Geometry check sheet. Reference: drawing and pictorial views, mm from the part's lowest x, y, z. A direction names the side the tool comes from. Round coordinates to 2 decimals unless told otherwise and drop trailing zeros. Write each loop counter-clockwise with the first axis right and the second up, starting at its lowest first coordinate (ties: lowest second). Pieces come first, ordered by that corner, then holes. Notation, with made-up numbers: (-1, 89.25) - (32, 89.25) arc R21 ccw to (32, 110.25) - close; hole circle Ø1 at (26, 42.25). An arc over 180 degrees is marked (long way). Use one line per item in the form item = value. Start each with the question number.
1) Draft check along Y on the marked faces 4, 5, 6 and 7. Enter one of: +Y half, -Y half, draft (parallel to the pull), parting line (faces both ways), or undercut.
2) Set-up check for the marked faces 1, 2 and 3: record each of +Z, -Z, +X, -X, +Y, -Y from which the full face is reachable in a straight line by a thin tool's end or side.
3) Section check B-B (x = 3.5). Record the boundary of the cut face in (y, z).
4) Section check D-D (y = 2.5). Record the boundary of the cut face in (x, z).
5) Gauge pin test, flat ends, axial feed: P1, Ø1.5, axis at y = 1.5, z = 1, coming from the +X side; P2, Ø2, axis at x = 1.5, y = 6.5, coming from the -Z side; P3, Ø0.8, axis at x = 6.5, z = 1, coming from the -Y side. Record the tip position at first contact, or that the pin passes through.
6) Section check A-A (z = 1.1). Record the boundary of the cut face in (x, y), then the cut area to 3 significant figures.
7) Section check C-C (y = 9). Record the boundary of the cut face in (x, z), then the cut area to 3 significant figures.
8) Scan lines: probe 1 along Y at (x, z) = (3.5, 2.25); probe 2 along Y at (x, z) = (4, 1.6); probe 3 along X at (y, z) = (8.75, 2.8). Record each from-to range of solid material in increasing order.
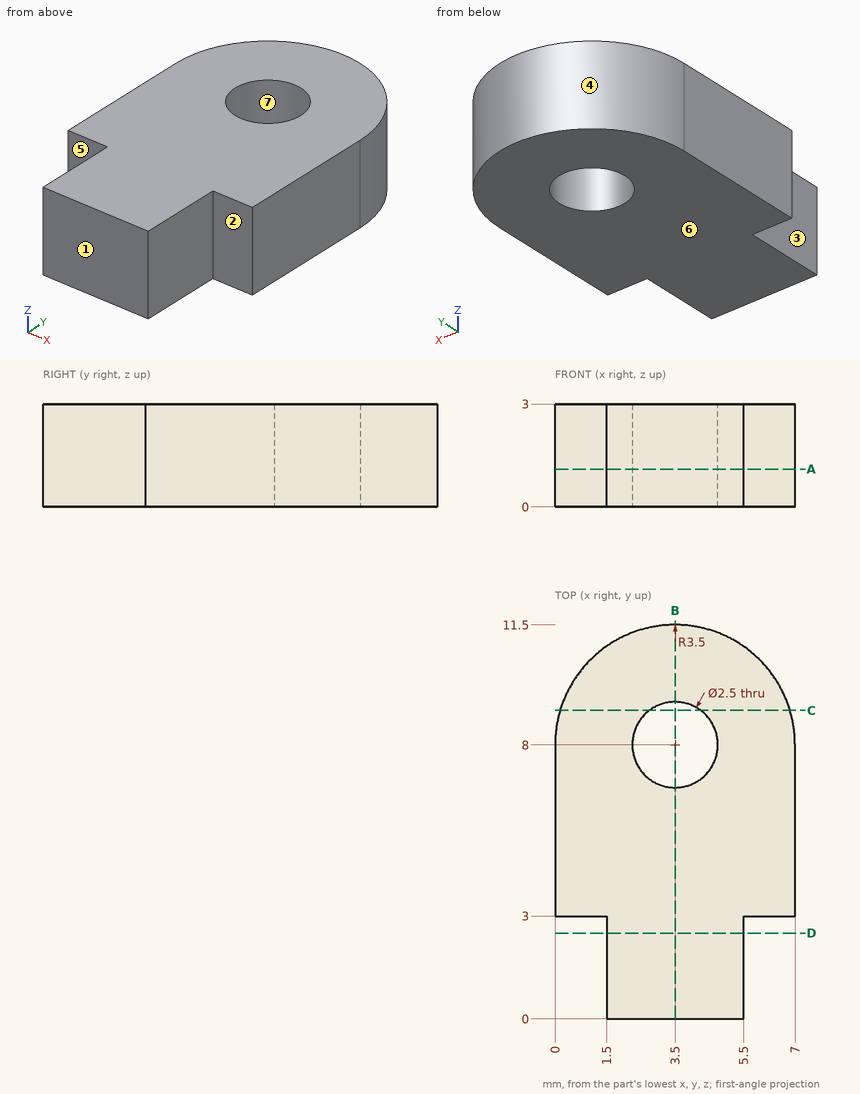
Results are:
q1.face_4 = +Y half
q1.face_5 = -Y half
q1.face_6 = draft
q1.face_7 = undercut
q2.face_1 = +Z, -Z, +X, -X, -Y
q2.face_2 = +Z, -Z, +X, -Y
q2.face_3 = +Z, -Z, -X, -Y
q3.outline = (0, 0) - (6.75, 0) - (6.75, 3) - (0, 3) - close; (9.25, 0) - (11.5, 0) - (11.5, 3) - (9.25, 3) - close
q4.outline = (1.5, 0) - (5.5, 0) - (5.5, 3) - (1.5, 3) - close
q5.P1 = 5.5
q5.P2 = 0
q5.P3 = 3
q6.outline = (0, 3) - (1.5, 3) - (1.5, 0) - (5.5, 0) - (5.5, 3) - (7, 3) - (7, 8) arc R3.5 ccw to (0, 8) - close; hole circle Ø2.5 at (3.5, 8)
q6.area = 61.3 mm²
q7.outline = (0.15, 0) - (2.75, 0) - (2.75, 3) - (0.15, 3) - close; (4.25, 0) - (6.85, 0) - (6.85, 3) - (4.25, 3) - close
q7.area = 15.6 mm²
q8.probe_1 = 0 to 6.75, 9.25 to 11.5
q8.probe_2 = 0 to 6.85, 9.15 to 11.46
q8.probe_3 = 0.08 to 2.5, 4.5 to 6.92
